Verification items for the finished model (mm, model axes). A direction names the side the tool comes from. Round coordinates to 2 decimals unless told otherwise and drop trailing zeros. Write each loop counter-clockwise with the first axis right and the second up, starting at its lowest first coordinate (ties: lowest second). Pieces come first, ordered by that corner, then holes. Notation, with made-up numbers: M 65,89.5 L 80,89.5 A18 ccw 80,93.5 Z; hole C 55,45 d7. An arc over 180 degrees is marked long. One line per item, written item: value. Start each with the question number.
Item 1: Section check A-A, the plane x = -10. Record the cut outline in (y, z), then the cut area to 3 significant figures.
Item 2: Tool access check on faces 1 (the face through (19, 0, 8.89)), 2 (the face through (-9, -7, 8.89)), 3 (the face through (26, 0, 2.247)). Record the directions out of +Z, -Z, +X, -X, +Y, -Y that give a thin tool (end or side, any length) a straight path to the whole face; none if there is none.
Item 3: Gauge pin test, flat ends, axial feed: pin 1 (4 mm diameter, centred on x = -5.84, z = 4, fed in from -Y); pin 2 (3 mm diameter, centred on x = 26, y = 0.5, fed in from -Z); pin 3 (2.5 mm diameter, centred on x = 12.5, z = 14.5, fed in from +Y). Record the tip position at first contact, or that the pin passes through.
Item 4: Draft check along Y on faces 4 (the face through (29.503, 0, 4)), 5 (the face through (14, 6.923, 14)), 6 (the face through (-10, -5.096, 5)). Enter one of: +Y half, -Y half, draft (parallel to the pull), parting line (faces both ways), or undercut.
Item 5: Section check B-B, the plane z = 8. Record the cut outline in (x, y), then the cut area to 3 significant figures.
Item 6: Thickness scan on probe 1 along Y at (x, z) = (-20, 3.25); probe 2 along X at (y, z) = (-10, 3.75); probe 3 along Z at (x, y) = (12.5, -9.5). Record the ranges inside material, lowest first. Write a range as from..to.
Item 7: Section check D-D, the plane x = -22. Record the cut outline in (y, z), then the cut area to 3 significant figures.
Item 8: Section check C-C, the plane y = 2. Record the cut outline in (x, z), then the cut area to 3 significant figures.
from build123d import *

# Parameters (mm, degrees)
F1_DEPTH = 7.5
F2_W     = 30.769231
F2_H     = 10.192308
F3_DEPTH = 8.891
F6_DEPTH = 8
F7_R     = 1.5
F8_DEPTH = 22.693308


with BuildPart() as f1:
    # F0 (on Front) → F1 (new body, symmetric)
    with BuildSketch(Plane.XZ):
        Polygon((-30.284615, 5.373077), (-48.846155, 5.373077), (-48.650771, 2.246923), (-30.284615, 2.246923), (-27.939999, 0), (20.515386, 0), (23.055386, 2.246923), (29.503077, 2.246923), (29.503077, 5.373077), (23.055386, 5.373077), (20.515386, 8.89), (-27.939999, 8.89), align=None)
    extrude(amount=F1_DEPTH, both=True)

    # F2 (on face) → F3 (cut, through all)
    with BuildSketch(Plane.XY.offset(8.89)):
        with Locations((-10, 0)):
            Rectangle(F2_W, F2_H)
    extrude(amount=-F3_DEPTH, mode=Mode.SUBTRACT)

    # F5 (on offset) → F6 (join)
    with BuildSketch(Plane.YZ.offset(10)):
        with BuildLine():
            ThreePointArc((-15.192308, 6.788462), (-14.020736, 3.960035), (-11.192308, 2.788462))
            Line((-11.192308, 2.788462), (11.192308, 2.788462))
            ThreePointArc((11.192308, 2.788462), (14.020736, 3.960035), (15.192308, 6.788462))
            Line((15.192308, 6.788462), (15.192308, 11.25))
            Line((15.192308, 11.25), (6.923077, 11.25))
            Line((6.923077, 11.25), (6.923077, 16.694458))
            ThreePointArc((6.923077, 16.694458), (0, 14.711539), (-6.923077, 16.694458))
            Line((-6.923077, 16.694458), (-6.923077, 11.25))
            Line((-6.923077, 11.25), (-15.192308, 11.25))
            Line((-15.192308, 11.25), (-15.192308, 6.788462))
        make_face()
    extrude(amount=F6_DEPTH)

    # F7 (on face) → F8 (cut, through all)
    with BuildSketch(Plane.XZ.offset(7.5)):
        with Locations((-21.837588, 4)):
            Circle(F7_R)
        with Locations((-13.837588, 4)):
            Circle(F7_R)
        with Locations((-5.837588, 4)):
            Circle(F7_R)
    extrude(amount=-F8_DEPTH, mode=Mode.SUBTRACT)


solid = f1.part
Response values:
1. outline: M -7.5,0 L -5.1,0 L -5.1,8.89 L -7.5,8.89 Z; M 5.1,0 L 7.5,0 L 7.5,8.89 L 5.1,8.89 Z
1. area: 42.7 mm2
2. face 1: +Z, +X, +Y, -Y
2. face 2: +Z, -X, +Y, -Y
2. face 3: -Z, +X, +Y, -Y
3. pin 1: stops at y = -7.5
3. pin 2: stops at z = 2.25
3. pin 3: stops at y = 6.92
4. face 4: draft
4. face 5: +Y half
4. face 6: undercut
5. outline: M -28.53,-7.5 L 10,-7.5 L 10,-15.19 L 18,-15.19 L 18,-7.5 L 21.16,-7.5 L 21.16,7.5 L 18,7.5 L 18,15.19 L 10,15.19 L 10,7.5 L -28.53,7.5 Z; hole M -25.38,-5.1 L 5.38,-5.1 L 5.38,5.1 L -25.38,5.1 Z
5. area: 555 mm2
6. probe 1: y = -7.5..-5.1, 5.1..7.5
6. probe 2: x = 10..18
6. probe 3: z = 2.79..11.25
7. outline: M -7.5,0 L -5.1,0 L -5.1,2.51 L -7.5,2.51 Z; M -7.5,5.49 L -5.1,5.49 L -5.1,8.89 L -7.5,8.89 Z; M 5.1,0 L 7.5,0 L 7.5,2.51 L 5.1,2.51 Z; M 5.1,5.49 L 7.5,5.49 L 7.5,8.89 L 5.1,8.89 Z
7. area: 28.4 mm2
8. outline: M -48.85,5.37 L -48.65,2.25 L -30.28,2.25 L -27.94,0 L -25.38,0 L -25.38,8.89 L -27.94,8.89 L -30.28,5.37 Z; M 5.38,0 L 20.52,0 L 23.06,2.25 L 29.5,2.25 L 29.5,5.37 L 23.06,5.37 L 20.52,8.89 L 18,8.89 L 18,14.87 L 10,14.87 L 10,8.89 L 5.38,8.89 Z
8. area: 312 mm2
